Can you work these out from the model? Positions are in its coordinate system, mm. Give positions to 0.01 mm unless a question says otherwise; leave off trailing zeros. Loops run counter-clockwise (first coordinate to the right, second up) from the corner with the lowest first, then second, coordinate; pieces in that order, holes last. Notation, with made-up numbers: (2, -28) - (15, -28) arc R19 cw to (15, -5) - close; hole circle Ø1 at (-22.5, 52.5). An arc over 180 degrees is marked (long way). Answer in a Markdown table with one row per item.
from build123d import *

# Parameters (mm, degrees)
SKETCH1_W           = 130
SKETCH1_H           = 100
EXTRUDE1_DEPTH      = 60
CUT_EXTRUDE1_DEPTH  = 61
CUT_EXTRUDE2_DEPTH  = 131
EXTRUDE2_DEPTH      = 15
EXTRUDE2_DEPTH_BACK = 55


with BuildPart() as part:
    # Sketch1 → Extrude1 (new body)
    with BuildSketch(Plane.XY):
        with Locations((65, 50)):
            Rectangle(SKETCH1_W, SKETCH1_H)
    extrude(amount=-EXTRUDE1_DEPTH)

    # Sketch2 → Cut-Extrude1 (cut, through all)
    with BuildSketch(Plane.XY):
        with BuildLine():
            Line((0, 65), (0, 111.499593367))
            Line((0, 111.499593367), (130, 111.499593367))
            Line((130, 111.499593367), (130, 65))
            ThreePointArc((130, 65), (65, 100), (0, 65))
        make_face()
    extrude(amount=-CUT_EXTRUDE1_DEPTH, mode=Mode.SUBTRACT)

    # Sketch3 → Cut-Extrude2 (cut, through all)
    with BuildSketch(Plane(origin=(130, 0, 0), x_dir=(0, 0, -1), z_dir=(1, 0, 0))):
        Polygon((0, 40), (60, 100), (0, 100), align=None)
    extrude(amount=-CUT_EXTRUDE2_DEPTH, mode=Mode.SUBTRACT)

    # Sketch4 → Extrude2 (add, two sides)
    with BuildSketch(Plane.XY) as extrude2_sk:
        with BuildLine():
            Line((40, 0), (90, 0))
            add(Edge.make_bspline(
                [(40, 0), (65, 150), (90, 0)],
                knots=[0, 0, 0, 1, 1, 1], degree=2))
        make_face()
    extrude(amount=EXTRUDE2_DEPTH)
    extrude(extrude2_sk.sketch, amount=-EXTRUDE2_DEPTH_BACK)


solid = part.part
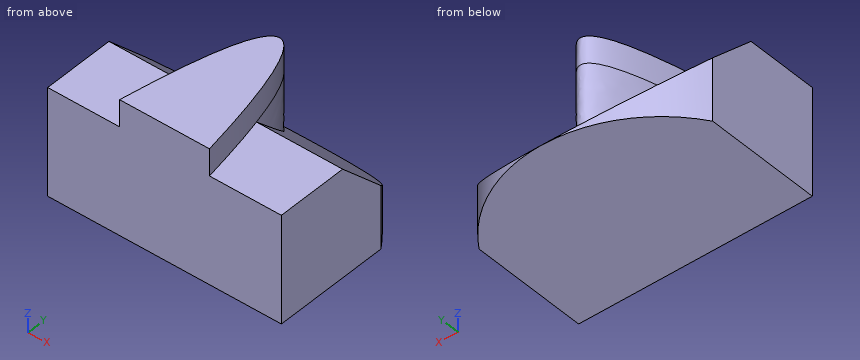
Q1. For pin 1 (20 mm diameter, centred on x = 111.5, y = 17, fed in from +Z); pin 2 (4 mm diameter, centred on y = 75.5, z = -19.5, fed in from -X); pin 3 (2 mm diameter, centred on x = 89, y = 54.5, fed in from +Z), each with a flat end and sliding along its axis, tell me the tip position at first contact or that it passes through.
Checked values:
| item | result |
|---|---|
| pin 1 | stops at z = 0 |
| pin 2 | stops at x = 61.46 |
| pin 3 | stops at z = -13.5 |
Q2. Imagine slicing it at A-A, the plane x = 30.5. Write out the boundary of the cut face in (y, z).
Checked values:
| item | result |
|---|---|
| outline | (0, -60) - (91.94, -60) - (91.94, -51.94) - (40, 0) - (0, 0) - close |
Q3. Imagine slicing it at B-B, the plane z = -39. Write out the boundary of the cut face in (x, y), and give its area (3 significant figures).
Checked values:
| item | result |
|---|---|
| outline | (0, 0) - (130, 0) - (130, 65) arc R77.86 ccw to (118.19, 79) - (11.81, 79) arc R77.86 ccw to (0, 65) - close |
| area | 10,100 mm² |
Q4. If I drill on line 1 (Z direction, x = 96.5, y = 39.5); line 2 (X direction, y = 74, z = -20); line 3 (X direction, y = 68.5, z = -41), over which ranges is the centre line in solid material (lowest first)? Write a range as [from, to].
Checked values:
| item | result |
|---|---|
| line 1 | z = [-60, 0] |
| line 2 | x = [62.11, 67.89] |
| line 3 | x = [2.45, 127.55] |
Q5. Imagine slicing it at D-D, the plane x = 97.5. Write out the boundary of the cut face in (y, z).
Checked values:
| item | result |
|---|---|
| outline | (0, -60) - (92.89, -60) - (92.89, -52.89) - (40, 0) - (0, 0) - close |
Q6. Imagine slicing it at C-C, the plane y = 78.5. Write out the boundary of the cut face in (x, z).
Checked values:
| item | result |
|---|---|
| outline | (11.28, -60) - (118.72, -60) - (118.72, -38.5) - (11.28, -38.5) - close |
